Geometry check sheet. Reference: drawing and pictorial views, mm from the part's lowest x, y, z. Round coordinates to 2 decimals unless told otherwise and drop trailing zeros. Write each loop counter-clockwise with the first axis right and the second up, starting at its lowest first coordinate (ties: lowest second). Pieces come first, ordered by that corner, then holes. Notation, with made-up numbers: M 29,27.5 L 57,27.5 A21 cw 57,37.5 Z; hole C 64.25,52 d5. An arc over 180 degrees is marked long. Answer in a Markdown table with one row per item.
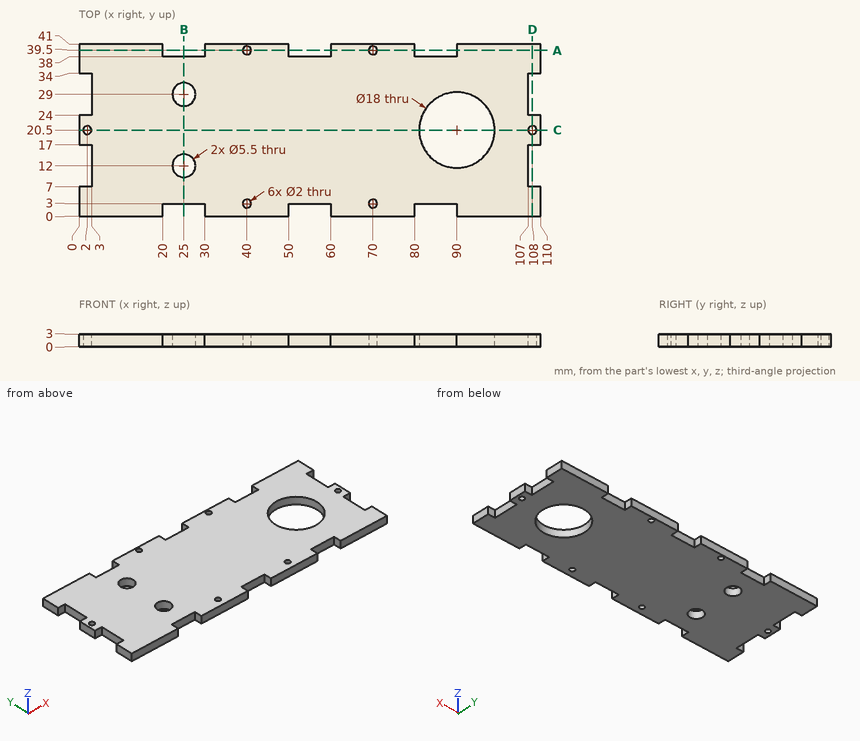
1. Section check A-A, the plane y = 39.5. Record the cut outline in (x, z), and give its area (3 significant figures).
Found:
| item | result |
|---|---|
| outline | M 0,0 L 20,0 L 20,3 L 0,3 Z; M 30,0 L 39,0 L 39,3 L 30,3 Z; M 41,0 L 50,0 L 50,3 L 41,3 Z; M 60,0 L 69,0 L 69,3 L 60,3 Z; M 71,0 L 80,0 L 80,3 L 71,3 Z; M 90,0 L 110,0 L 110,3 L 90,3 Z |
| area | 228 mm2 |
2. Go/stop test with flat-tipped pins: pin 1 (4 mm diameter, centred on x = 73.5, y = 24.5, fed in from -Z); pin 2 (1 mm diameter, centred on y = 31.5, z = 0.5, fed in from -X). Record where each tip stops, or that it passes through.
Found:
| item | result |
|---|---|
| pin 1 | stops at z = 0 |
| pin 2 | stops at x = 3 |
3. Section check B-B, the plane x = 25. Record the cut outline in (y, z).
Found:
| item | result |
|---|---|
| outline | M 3,0 L 9.25,0 L 9.25,3 L 3,3 Z; M 14.75,0 L 26.25,0 L 26.25,3 L 14.75,3 Z; M 31.75,0 L 38,0 L 38,3 L 31.75,3 Z |
4. Scan lines: L1, parallel to Y at x = 70, z = 0.6; L2, parallel to Y at x = 25.5, z = 1; L3, parallel to X at y = 7.5, z = 0.5. Record each from-to range of solid material in increasing order.
Found:
| item | result |
|---|---|
| L1 | y = 0 to 2, 4 to 38.5, 40.5 to 41 |
| L2 | y = 3 to 9.3, 14.7 to 26.3, 31.7 to 38 |
| L3 | x = 3 to 107 |
5. Section check C-C, the plane y = 20.5. Record the cut outline in (x, z), and give its area (3 significant figures).
Found:
| item | result |
|---|---|
| outline | M 0,0 L 1,0 L 1,3 L 0,3 Z; M 3,0 L 81,0 L 81,3 L 3,3 Z; M 99,0 L 107,0 L 107,3 L 99,3 Z; M 109,0 L 110,0 L 110,3 L 109,3 Z |
| area | 264 mm2 |
6. Section check D-D, the plane x = 108. Record the cut outline in (y, z).
Found:
| item | result |
|---|---|
| outline | M 0,0 L 7,0 L 7,3 L 0,3 Z; M 17,0 L 19.5,0 L 19.5,3 L 17,3 Z; M 21.5,0 L 24,0 L 24,3 L 21.5,3 Z; M 34,0 L 41,0 L 41,3 L 34,3 Z |
